Could you check a few things on this model? Use its own coordinates, in mm. Give positions to 0.01 mm unless a question says otherwise; leave off trailing zeros. Loops run counter-clockwise (first coordinate to the right, second up) from the corner with the lowest first, then second, coordinate; pieces in that order, holes last. Notation, with made-up numbers: M -23.5,80.5 L 5.5,80.5 A16 ccw 5.5,108.5 Z; hole C 6.5,26 d11. An arc over 180 degrees is marked long. Return JSON: item names as keys, results as strings. Group by question number.
1. If we section it at C-C (y = 2.3): Write out the boundary of the cut face in (x, z).
2. If we section it at A-A (x = 0): Write out the boundary of the cut face in (y, z) (1 decimal).
3. Please list where these lines run through material, in increasing order: line 1 (X direction, y = 1.55, z = 0); line 2 (X direction, y = 1.7, z = 0); line 3 (Y direction, x = 12, z = -21.5).
4. For pin 1 (4 mm diameter, centred on x = 4, z = -19, fed in from -Y); pin 2 (2 mm diameter, centred on x = 20, z = -15, fed in from +Y); pin 3 (1 mm diameter, centred on y = 0.5, z = -20, fed in from +X), each with a flat end and sliding along its axis, tell me the tip position at first contact or that it passes through.
5. If we section it at B-B (z = 0): Write out the boundary of the cut face in (x, y) (1 decimal).
6. If we section it at D-D (z = -5.5): Write out the boundary of the cut face in (x, y) (1 decimal), plus the area to 3 significant figures.
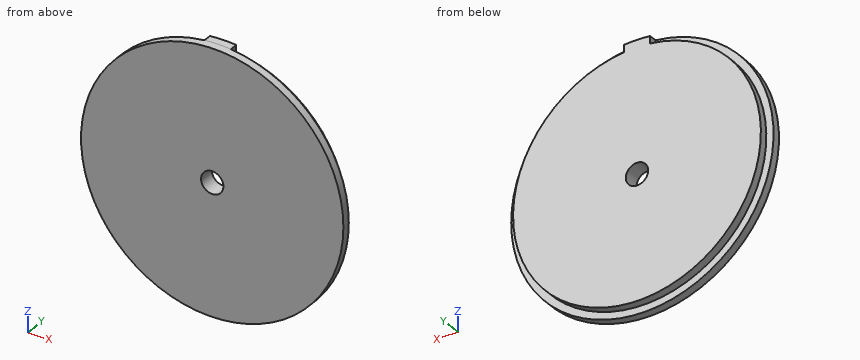
```python
from build123d import *

# Parameters (mm, degrees)
SKETCH1_R                 = 25.273
BOSS_EXTRUDE1_DEPTH       = 1.5875
SKETCH2_R                 = 23.876
BOSS_EXTRUDE2_DEPTH       = 1.5875
BOSS_EXTRUDE3_DEPTH       = 1.5875
F_8_CLEARANCE_HOLE1_D     = 4.3053
F_8_CLEARANCE_HOLE1_DEPTH = 3.175


with BuildPart() as part:
    # Sketch1 → Boss-Extrude1 (new body)
    with BuildSketch(Plane(origin=(0, 0, 0), x_dir=(1, 0, 0), z_dir=(0, 1, 0))):
        Circle(SKETCH1_R)
    extrude(amount=BOSS_EXTRUDE1_DEPTH)

    # Sketch2 → Boss-Extrude2 (add)
    with BuildSketch(Plane(origin=(0, 1.5875, 0), x_dir=(1, 0, 0), z_dir=(0, 1, 0))):
        Circle(SKETCH2_R)
    extrude(amount=BOSS_EXTRUDE2_DEPTH)

    # Sketch3 → Boss-Extrude3 (add)
    with BuildSketch(Plane(origin=(0, 1.5875, 0), x_dir=(1, 0, 0), z_dir=(0, 1, 0))):
        with BuildLine():
            Line((-2.54, -25.14503786), (-2.54, -23.740509177))
            ThreePointArc((-2.54, -23.740509177), (0, -23.876), (2.54, -23.740509177))
            Line((2.54, -23.740509177), (2.54, -25.14503786))
            ThreePointArc((2.54, -25.14503786), (0, -25.273), (-2.54, -25.14503786))
        make_face()
    extrude(amount=BOSS_EXTRUDE3_DEPTH)

    # #8 Clearance Hole1
    with Locations(Plane.ZX.offset(3.175)):
        with Locations((0, 0)):
            Hole(F_8_CLEARANCE_HOLE1_D / 2, depth=F_8_CLEARANCE_HOLE1_DEPTH)


solid = part.part
```
Answer:
{
 "1": {"outline": "M -2.54,23.74 A23.88 ccw long 2.54,23.74 L 2.54,25.15 A25.27 ccw -2.54,25.15 Z; hole C 0,0 d4.31"},
 "2": {"outline": "M 0,-25.3 L 1.6,-25.3 L 1.6,-23.9 L 3.2,-23.9 L 3.2,-2.2 L 0,-2.2 Z; M 0,2.2 L 3.2,2.2 L 3.2,25.3 L 0,25.3 Z"},
 "3": {"line 1": "x = -25.27 to -2.15, 2.15 to 25.27", "line 2": "x = -23.88 to -2.15, 2.15 to 23.88", "line 3": "y = 0 to 1.59"},
 "4": {"pin 1": "stops at y = 0", "pin 2": "stops at y = 1.59", "pin 3": "stops at x = 16.08"},
 "5": {"outline": "M -25.3,0 L -2.2,0 L -2.2,3.2 L -23.9,3.2 L -23.9,1.6 L -25.3,1.6 Z; M 2.2,0 L 25.3,0 L 25.3,1.6 L 23.9,1.6 L 23.9,3.2 L 2.2,3.2 Z"},
 "6": {"outline": "M -24.7,0 L 24.7,0 L 24.7,1.6 L 23.2,1.6 L 23.2,3.2 L -23.2,3.2 L -23.2,1.6 L -24.7,1.6 Z", "area": "152 mm²"}
}
